```python
from build123d import *

# Parameters (mm, degrees)
SKETCH1_R           = 3.175
BOSS_EXTRUDE1_DEPTH = 38.1
SKETCH2_W           = 22.86
SKETCH2_H           = 20.32
CUT_EXTRUDE1_DEPTH  = 25.4
SKETCH3_R           = 3.175
CUT_EXTRUDE2_DEPTH  = 25.4


with BuildPart() as part:
    # Sketch1 → Boss-Extrude1 (new body)
    with BuildSketch(Plane(origin=(0, 0, 0), x_dir=(0, 0, -1), z_dir=(1, 0, 0))):
        with BuildLine():
            Line((-6.35, 0), (6.35, 0))
            Line((6.35, 0), (6.35, 20.32))
            ThreePointArc((6.35, 20.32), (0, 26.67), (-6.35, 20.32))
            Line((-6.35, 20.32), (-6.35, 0))
        make_face()
        with Locations(Location((0, 20.32, 0), (0, 0, 180))):
            Circle(SKETCH1_R, mode=Mode.SUBTRACT)
    extrude(amount=BOSS_EXTRUDE1_DEPTH)

    # Sketch2 → Cut-Extrude1 (cut)
    with BuildSketch(Plane.XY.offset(6.35)):
        with Locations((19.05, 16.51)):
            Rectangle(SKETCH2_W, SKETCH2_H)
    extrude(amount=-CUT_EXTRUDE1_DEPTH, mode=Mode.SUBTRACT)

    # Sketch3 → Cut-Extrude2 (cut)
    with BuildSketch(Plane(origin=(0, 6.35, 0), x_dir=(1, 0, 0), z_dir=(0, 1, 0))):
        with Locations(Location((19.05, 0, 0), (0, 0, 180))):
            Circle(SKETCH3_R)
    extrude(amount=-CUT_EXTRUDE2_DEPTH, mode=Mode.SUBTRACT)


solid = part.part
```
Model file for the job. Use its own axes, mm. A direction names the side the tool comes from. Coordinates: 2 decimals unless noted, no trailing zeros. Write each loop counter-clockwise with the first axis right and the second up, starting at its lowest first coordinate (ties: lowest second). Pieces come first, ordered by that corner, then holes. Notation, with made-up numbers: (85.5, 5) - (123.5, 5) arc R30 ccw to (123.5, 43) - close; hole circle Ø1 at (-22.75, -24). An arc over 180 degrees is marked (long way). Use a Markdown table: item, result. Add a question column.
Item 1: Band-saw the part on B-B, the plane y = 10.25. Write the cut outline in (x, z), and give its area (3 significant figures).
Item 2: Two-plate mould, pull along X, no slides. Class faces 1 (the face through (0, 11, 0)), 2 (the face through (23, 0, 0)), 3 (the face through (30.48, 14, 0)), 4 (the face through (16.02, 3.22, 0.95)): pulls with the +X half, pulls with the -X half, needs draft (parallel to the pull), parting line crosses it, or undercut.
Item 3: Band-saw the part on A-A, the plane x = 19.05. Write the cut outline in (y, z) (3 decimals).
Item 4: 3-axis set-ups, long thin cutter, end or side, ignore diameter. For faces 5 (the face through (19, 6, -6.35)), 6 (the face through (7.62, 14, 0)): which of +Z, -Z, +X, -X, +Y, -Y reach the whole face in a straight line?
Item 5: Drop a flat-ended pin along its axis: pin 1 (4 mm diameter, centred on x = 24.5, z = -2, fed in from +Y). Give the stop position or say it passes through.
Item 6: Drill centre lines: line 1 along Y through (x, z) = (33.5, 0) (3 decimals); line 2 along Z through (x, y) = (3.75, 20.32) (3 decimals); line 3 along X through (y, z) = (10.75, -0.5). Where is each one in solid material? Low to high.
Item 7: Band-saw the part on C-C, the plane z = 0. Write the cut outline in (x, y) (3 decimals), and give its area (3 significant figures).
Item 8: Band-saw the part on D-D, the plane y = 18. Write the cut outline in (x, z).
A:
| question | item | result |
|---|---|---|
| 1 | outline | (0, -6.35) - (7.62, -6.35) - (7.62, 6.35) - (0, 6.35) - close; (30.48, -6.35) - (38.1, -6.35) - (38.1, 6.35) - (30.48, 6.35) - close |
| 1 | area | 194 mm² |
| 2 | face 1 | pulls with the -X half |
| 2 | face 2 | needs draft |
| 2 | face 3 | undercut |
| 2 | face 4 | undercut |
| 3 | outline | (0, -6.35) - (6.35, -6.35) - (6.35, -3.175) - (0, -3.175) - close; (0, 3.175) - (6.35, 3.175) - (6.35, 6.35) - (0, 6.35) - close |
| 4 | face 5 | -Z, +X, -X, +Y, -Y |
| 4 | face 6 | +Z, -Z, +Y |
| 5 | pin 1 | stops at y = 6.35 |
| 6 | line 1 | y = 0 to 17.145, 23.495 to 26.67 |
| 6 | line 2 | z = -6.35 to -3.175, 3.175 to 6.35 |
| 6 | line 3 | x = 0 to 7.62, 30.48 to 38.1 |
| 7 | outline | (0, 0) - (15.875, 0) - (15.875, 6.35) - (7.62, 6.35) - (7.62, 17.145) - (0, 17.145) - close; (0, 23.495) - (7.62, 23.495) - (7.62, 26.67) - (0, 26.67) - close; (22.225, 0) - (38.1, 0) - (38.1, 17.145) - (30.48, 17.145) - (30.48, 6.35) - (22.225, 6.35) - close; (30.48, 23.495) - (38.1, 23.495) - (38.1, 26.67) - (30.48, 26.67) - close |
| 7 | area | 415 mm² |
| 8 | outline | (0, -6.35) - (7.62, -6.35) - (7.62, -2.17) - (0, -2.17) - close; (0, 2.17) - (7.62, 2.17) - (7.62, 6.35) - (0, 6.35) - close; (30.48, -6.35) - (38.1, -6.35) - (38.1, -2.17) - (30.48, -2.17) - close; (30.48, 2.17) - (38.1, 2.17) - (38.1, 6.35) - (30.48, 6.35) - close |
